The model under review builds one solid part; all positions refer to its coordinate system, in mm. Face numbers are marked on the shaded views. A direction names the side the tool comes from. Round coordinates to 2 decimals unless told otherwise and drop trailing zeros. Order: outer loops, then holes, each group sorted by start corner. A loop starts at its lowest first (then second) coordinate and runs counter-clockwise, first axis right, second up. Notation, with made-up numbers: (-9, 68.25) -> (16, 68.25) arc R25 cw to (16, 83.25) -> close; hole circle Ø10 at (4.25, -28.5). An arc over 180 degrees is marked (long way). Use a Markdown table: item, result. Add a question column.
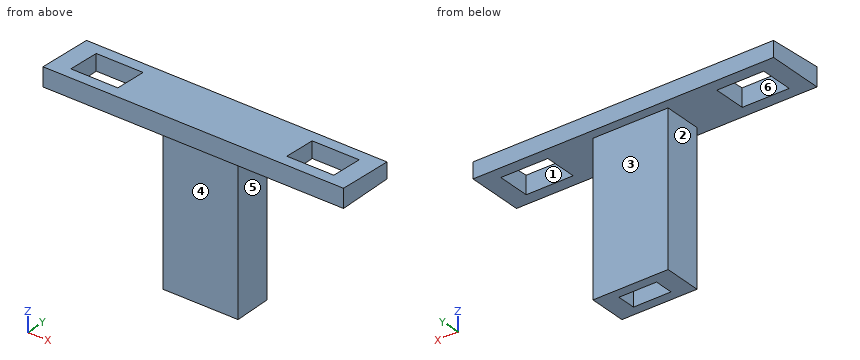
```python
from build123d import *

# Parameters (mm, degrees)
F0_W     = 101.6
F0_H     = 19.05
F1_DEPTH = 6.35
F2_W     = 15.875
F2_H     = 11.1125
F3_DEPTH = 6.35
F4_W     = 15.875
F4_H     = 11.1125
F5_DEPTH = 6.35
F7_DEPTH = 101.6
F8_W     = 25.4
F8_H     = 12.7
F8_W_2   = 12.7
F8_H_2   = 6.35
F9_DEPTH = 50.8


with BuildPart() as f1:
    # F0 (on Top) → F1 (new body)
    with BuildSketch(Plane.XY):
        Rectangle(F0_W, F0_H)
    extrude(amount=F1_DEPTH)

    # F2 (on face) → F3 (cut)
    with BuildSketch(Plane.XY.offset(6.35)):
        with Locations((-36.5125, 0)):
            Rectangle(F2_W, F2_H)
    extrude(amount=-F3_DEPTH, mode=Mode.SUBTRACT)

    # F4 (on face) → F5 (cut)
    with BuildSketch(Plane.XY.offset(6.35)):
        with Locations((36.5125, 0)):
            Rectangle(F4_W, F4_H)
    extrude(amount=-F5_DEPTH, mode=Mode.SUBTRACT)

    # F6 (on face) → F7 (cut)
    with BuildSketch(Plane.YZ.offset(50.8)):
        Polygon((9.525, 6.35), (-9.525, 6.35), (9.525, 5.351632), align=None)
    extrude(amount=-F7_DEPTH, mode=Mode.SUBTRACT)

    # F8 (on face) → F9 (join)
    with BuildSketch(Plane(origin=(0, 0, 0), x_dir=(1, 0, 0), z_dir=(0, 0, -1))):
        Rectangle(F8_W, F8_H)
        Rectangle(F8_W_2, F8_H_2, mode=Mode.SUBTRACT)
    extrude(amount=F9_DEPTH)


solid = f1.part
```
Q1. To check wall thickness, follow line 1 along X through (y, z) = (1.75, 2) (3 decimals); line 2 along X through (y, z) = (-1.25, -28.5); line 3 along Y through (x, z) = (-5, -43) (3 decimals). State the ranges of each line that lie inside material, in increasing order.
Q2. Add section D-D, the plane y = -0.25. Give the boundary of the cut face in (x, z) (3 decimals).
Q3. Add section C-C, the plane x = -34. Give the boundary of the cut face in (y, z) (3 decimals).
Q4. For the marked faces 1, 2 and 3, list the 3-axis set-ups (+Z, -Z, +X, -X, +Y, -Y) from which the entire face can be reached by the end or side of a thin tool; tool diameter is ignored.
Q5. Draft analysis for pull direction X (two halves, no side actions). For the marked faces 4, 5 and 6, state which applies: released by +X, released by -X, zero draft, split by the parting line, or undercut.
Q6. Add section A-A, the plane z = -1. Give the boundary of the cut face in (x, y) (3 decimals), then the cut area to 3 significant figures.
Q7. Add section B-B, the plane x = 3.5. Give the boundary of the cut face in (y, z) (3 decimals), then the cut area to 3 significant figures.
Q8. For pin 1 (12 mm diameter, centred on x = -11, z = -38, fed in from -Y); pin 2 (6 mm diameter, centred on y = 7, z = -24.5, fed in from +X); pin 3 (5 mm diameter, centred on x = 17, z = -33.5, fed in from -Y); pin 4 (1.9 mm diameter, centred on y = 0.5, z = -29, fed in from -X), all flat-tipped, find the tip position at first contact; note any pin that passes through.
Return value:
| question | item | result |
|---|---|---|
| 1 | line 1 | -50.8 to -44.45, -28.575 to 28.575, 44.45 to 50.8 |
| 1 | line 2 | -12.7 to -6.35, 6.35 to 12.7 |
| 1 | line 3 | -6.35 to -3.175, 3.175 to 6.35 |
| 2 | outline | (-50.8, 0) -> (-44.45, 0) -> (-44.45, 5.864) -> (-50.8, 5.864) -> close; (-28.575, 0) -> (-12.7, 0) -> (-12.7, -50.8) -> (-6.35, -50.8) -> (-6.35, 0) -> (6.35, 0) -> (6.35, -50.8) -> (12.7, -50.8) -> (12.7, 0) -> (28.575, 0) -> (28.575, 5.864) -> (-28.575, 5.864) -> close; (44.45, 0) -> (50.8, 0) -> (50.8, 5.864) -> (44.45, 5.864) -> close |
| 3 | outline | (-9.525, 0) -> (-5.556, 0) -> (-5.556, 6.142) -> (-9.525, 6.35) -> close; (5.556, 0) -> (9.525, 0) -> (9.525, 5.352) -> (5.556, 5.56) -> close |
| 4 | face 1 | +Z, -Z |
| 4 | face 2 | -Z, -X, +Y, -Y |
| 4 | face 3 | -Z, +X, -X, +Y |
| 5 | face 4 | zero draft |
| 5 | face 5 | released by +X |
| 5 | face 6 | undercut |
| 6 | outline | (-12.7, -6.35) -> (12.7, -6.35) -> (12.7, 6.35) -> (-12.7, 6.35) -> close; hole (-6.35, -3.175) -> (6.35, -3.175) -> (6.35, 3.175) -> (-6.35, 3.175) -> close |
| 6 | area | 242 mm² |
| 7 | outline | (-9.525, 0) -> (-6.35, 0) -> (-6.35, -50.8) -> (-3.175, -50.8) -> (-3.175, 0) -> (3.175, 0) -> (3.175, -50.8) -> (6.35, -50.8) -> (6.35, 0) -> (9.525, 0) -> (9.525, 5.352) -> (-9.525, 6.35) -> close |
| 7 | area | 434 mm² |
| 8 | pin 1 | y = -6.35 |
| 8 | pin 2 | x = 12.7 |
| 8 | pin 3 | through |
| 8 | pin 4 | x = -12.7 |
